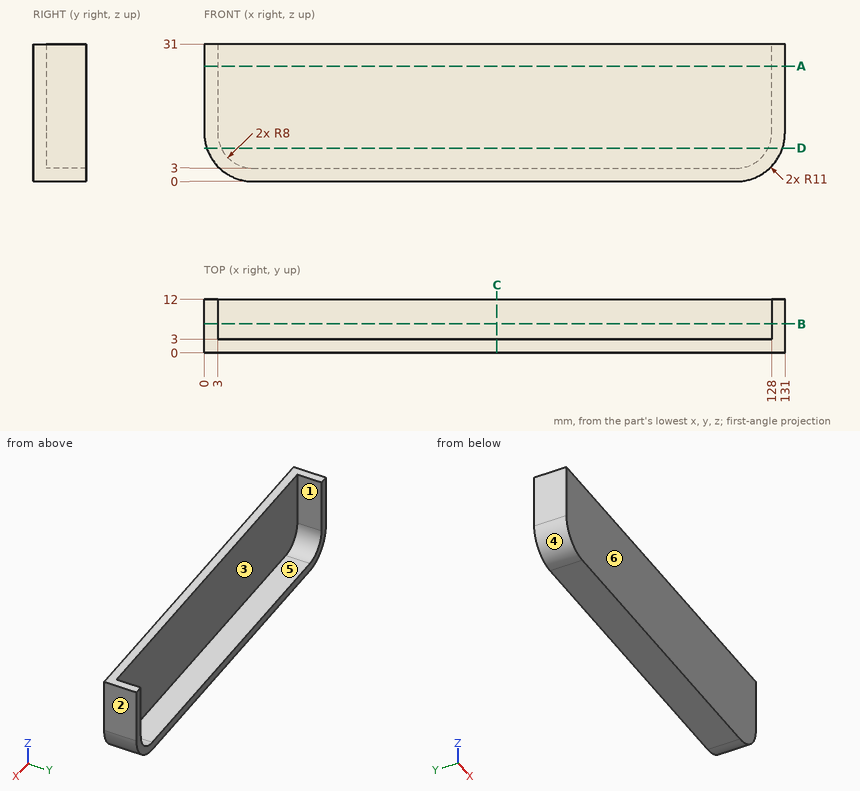
Check sheet for the drawn part. Datum: minimum x, y, z corner. Units: mm. A direction names the side the tool comes from. Round coordinates to 2 decimals unless told otherwise and drop trailing zeros. Order: outer loops, then holes, each group sorted by start corner. A loop starts at its lowest first (then second) coordinate and runs counter-clockwise, first axis right, second up.
1. Thickness scan on L1, parallel to X at y = 10, z = 29; L2, parallel to Z at x = 47, y = 10.5. Record the ranges inside material, lowest first.
Final values:
L1: x = 0 to 3, 128 to 131
L2: z = 0 to 3
2. Section check B-B on y = 6.5. Record the cut outline in (x, z).
Final values:
outline: (0, 11) arc R11 ccw to (11, 0) - (120, 0) arc R11 ccw to (131, 11) - (131, 31) - (128, 31) - (128, 11) arc R8 cw to (120, 3) - (11, 3) arc R8 cw to (3, 11) - (3, 31) - (0, 31) - close
3. Section check D-D on z = 7.5. Record the cut outline in (x, y), then the cut area to 3 significant figures.
Final values:
outline: (0.57, 0) - (130.43, 0) - (130.43, 12) - (127.19, 12) - (127.19, 3) - (3.81, 3) - (3.81, 12) - (0.57, 12) - close
area: 448 mm2
4. Section check C-C on x = 66. Record the cut outline in (y, z).
Final values:
outline: (0, 0) - (12, 0) - (12, 3) - (3, 3) - (3, 31) - (0, 31) - close
5. Section check A-A on z = 26. Record the cut outline in (x, y).
Final values:
outline: (0, 0) - (131, 0) - (131, 12) - (128, 12) - (128, 3) - (3, 3) - (3, 12) - (0, 12) - close
6. Access from +Z, -Z, +X, -X, +Y, -Y to the whole of each face (thin tool, end or side, straight path). Record for the marked faces 5 and 6.
Final values:
face 5: +Z, +Y
face 6: +Z, -Z, +X, -X, -Y
7. Go/stop test with flat-tipped pins: P1, Ø5, axis at y = 9.5, z = 8, coming from the -X side; P2, Ø6, axis at x = 24.5, z = 17.5, coming from the +Y side; P3, Ø4.5, axis at x = 45, y = 7, coming from the +Z side. Record where each tip stops, or that it passes through.
Final values:
P1: stops at x = 0.01
P2: stops at y = 3
P3: stops at z = 3
8. Release check for a two-part mould opening along X. For the marked faces 1, 2, 3 and 4 record: +X half, -X half, draft (parallel to the pull), parting line (faces both ways), or undercut.
Final values:
face 1: undercut
face 2: +X half
face 3: undercut
face 4: -X half
